```python
from build123d import *

# Parameters (mm, degrees)
SKETCH1_W               = 71
SKETCH1_H               = 70
SKETCH1_W_2             = 68
SKETCH1_H_2             = 67
BOSS_EXTRUDE1_DEPTH     = 17.2
BOSS_EXTRUDE2_START     = 17.2
SKETCH1_2_W             = 71
SKETCH1_2_H             = 70
BOSS_EXTRUDE2_DEPTH     = 1.5
CUT_EXTRUDE1_REACH      = 96.232
SKETCH6_W               = 5.15
SKETCH6_H               = 1.8
MIRROR2_COPY_1_REACH    = 96.232
MIRROR2_COPY_1_SKETCH_W = 5.15
MIRROR2_COPY_1_SKETCH_H = 1.8
CUT_EXTRUDE2_REACH      = 96.978
SKETCH7_W               = 9.92
SKETCH7_H               = 21.65
SKETCH8_R               = 2.15
SKETCH8_R_2             = 0.4
SKETCH8_W               = 1.5
SKETCH8_H               = 1.5
BOSS_EXTRUDE6_DEPTH     = 5.7


with BuildPart() as part:
    # Sketch1 → Boss-Extrude1 (new body)
    with BuildSketch(Plane.XY):
        with Locations((-24.75, 25.25)):
            Rectangle(SKETCH1_W, SKETCH1_H)
        with Locations((-24.75, 25.25)):
            Rectangle(SKETCH1_W_2, SKETCH1_H_2, mode=Mode.SUBTRACT)
    extrude(amount=BOSS_EXTRUDE1_DEPTH)

    # Sketch1<2> → Boss-Extrude2 (add)
    with BuildSketch(Plane.XY.offset(BOSS_EXTRUDE2_START)):
        with Locations((-24.75, 25.25)):
            Rectangle(SKETCH1_2_W, SKETCH1_2_H)
    extrude(amount=BOSS_EXTRUDE2_DEPTH)

    # Sketch6 → Cut-Extrude1 (cut, up to next)
    with BuildSketch(Plane(origin=(0, 60.25, 0), x_dir=(1, 0, 0), z_dir=(0, 1, 0)), mode=Mode.PRIVATE) as cut_extrude1_sk1:
        with Locations((6.675, -5.25)):
            Rectangle(SKETCH6_W, SKETCH6_H)
    cut_extrude1_tool1 = extrude(cut_extrude1_sk1.sketch, amount=-CUT_EXTRUDE1_REACH, mode=Mode.PRIVATE) & part.part
    cut_extrude1 = cut_extrude1_tool1.solids().sort_by_distance((6.675, 60.25, 5.25))[0]
    add(cut_extrude1, mode=Mode.SUBTRACT)

    # Mirror1: Cut-Extrude1 across plane
    add(cut_extrude1.mirror(Plane(origin=(-24.75, 0, 0), x_dir=(0, 0, 1), z_dir=(1, 0, 0))), mode=Mode.SUBTRACT)

    # Mirror2: Cut-Extrude1 across plane
    add(cut_extrude1.mirror(Plane.ZX.offset(25.25)), mode=Mode.SUBTRACT)

    # Mirror2 copy 1 sketch → Mirror2 copy 1 (cut, up to next)
    with BuildSketch(Plane(origin=(-49.5, -9.75, 0), x_dir=(-1, 0, 0), z_dir=(0, -1, 0)), mode=Mode.PRIVATE) as mirror2_copy_1_sk1:
        with Locations((6.675, -5.25)):
            Rectangle(MIRROR2_COPY_1_SKETCH_W, MIRROR2_COPY_1_SKETCH_H)
    mirror2_copy_1_tool1 = extrude(mirror2_copy_1_sk1.sketch, amount=-MIRROR2_COPY_1_REACH, mode=Mode.PRIVATE) & part.part
    add(mirror2_copy_1_tool1.solids().sort_by_distance((-56.175, -9.75, 5.25))[0], mode=Mode.SUBTRACT)

    # Sketch7 → Cut-Extrude2 (cut, up to next)
    with BuildSketch(Plane.ZY.offset(60.25), mode=Mode.PRIVATE) as cut_extrude2_sk1:
        with Locations((6.74, 22.95)):
            Rectangle(SKETCH7_W, SKETCH7_H)
    cut_extrude2_tool1 = extrude(cut_extrude2_sk1.sketch, amount=-CUT_EXTRUDE2_REACH, mode=Mode.PRIVATE) & part.part
    add(cut_extrude2_tool1.solids().sort_by_distance((-60.25, 22.95, 6.74))[0], mode=Mode.SUBTRACT)

    # Sketch8 → Boss-Extrude6 (add)
    # profile 1 of 4: a face of its own
    with BuildSketch(Plane(origin=(0, 0, 17.2), x_dir=(-1, 0, 0), z_dir=(0, 0, -1))):
        with Locations((51.65, 49.525)):
            Circle(SKETCH8_R)
        with Locations((51.65, 49.525)):
            Circle(SKETCH8_R_2, mode=Mode.SUBTRACT)
    # profile 2 of 4: a face of its own
    with BuildSketch(Plane(origin=(0, 0, 17.2), x_dir=(-1, 0, 0), z_dir=(0, 0, -1))):
        with Locations((-2.3, 49.625)):
            Circle(SKETCH8_R)
        with Locations((-2.3, 49.625)):
            Circle(SKETCH8_R_2, mode=Mode.SUBTRACT)
    # profile 3 of 4: a face of its own
    with BuildSketch(Plane(origin=(0, 0, 17.2), x_dir=(-1, 0, 0), z_dir=(0, 0, -1))):
        with Locations((-1.95, 1.075)):
            Circle(SKETCH8_R)
        with Locations((-1.95, 1.075)):
            Circle(SKETCH8_R_2, mode=Mode.SUBTRACT)
    # profile 4 of 4: a face of its own
    with BuildSketch(Plane(origin=(0, 0, 17.2), x_dir=(-1, 0, 0), z_dir=(0, 0, -1))):
        with Locations((53, -0.125)):
            Rectangle(SKETCH8_W, SKETCH8_H)
    extrude(amount=BOSS_EXTRUDE6_DEPTH)


solid = part.part
```
For this review, take the finished solid that the model builds, in its own axes (mm). A direction names the side the tool comes from. Coordinates: 2 decimals unless noted, no trailing zeros. Order: outer loops, then holes, each group sorted by start corner. A loop starts at its lowest first (then second) coordinate and runs counter-clockwise, first axis right, second up. Notation, with made-up numbers: (26, 49) -> (60, 49) arc R13 cw to (60, 67) -> close; hole circle Ø8 at (36, 75.5). An arc over 180 degrees is marked (long way). Answer as CSV lines item,"result".
Q1. We need section C-C (z = 14.75). Count the separate pieces of the cut face and the enclosed holes in it, plus the area to 3 significant figures.
Model answer:
separate pieces,"5"
enclosed holes,"4"
area,"458 mm2"
Q2. Draft analysis for pull direction Y (two halves, no side actions). For faces 3 (the face through (10.75, 25, 9)), 4 (the face through (2.5, 1.1, 11.5)), 5 (the face through (1.144, 51.438, 14.39)), 6 (the face through (-25, 60.25, 9)), state which applies: released by +Y, released by -Y, zero draft, split by the parting line, or undercut.
Model answer:
face 3,"zero draft"
face 4,"undercut"
face 5,"undercut"
face 6,"released by +Y"
Q3. Clearance check with flat-ended pins moving along their axes: pin 1 Ø20 at (x, y) = (-26, 20) entering from -Z; pin 2 Ø1.6 at (x, y) = (-52.5, 0) entering from -Z. State where each tip first meets the part, or that it passes through.
Model answer:
pin 1,"stops at z = 17.2"
pin 2,"stops at z = 11.5"
Q4. We need section A-A (x = -55). State the section outline as (y, z) points, plus the area to 3 significant figures.
Model answer:
outline,"(-9.75, 0) -> (-8.25, 0) -> (-8.25, 4.35) -> (-9.75, 4.35) -> close; (-9.75, 6.15) -> (-8.25, 6.15) -> (-8.25, 17.2) -> (58.75, 17.2) -> (58.75, 6.15) -> (60.25, 6.15) -> (60.25, 18.7) -> (-9.75, 18.7) -> close; (58.75, 0) -> (60.25, 0) -> (60.25, 4.35) -> (58.75, 4.35) -> close"
area,"151 mm2"
Q5. We need section B-B (y = 21). State the section outline as (x, z) points, plus the area to 3 significant figures.
Model answer:
outline,"(-60.25, 0) -> (-58.75, 0) -> (-58.75, 1.78) -> (-60.25, 1.78) -> close; (-60.25, 11.7) -> (-58.75, 11.7) -> (-58.75, 17.2) -> (9.25, 17.2) -> (9.25, 0) -> (10.75, 0) -> (10.75, 18.7) -> (-60.25, 18.7) -> close"
area,"143 mm2"
Q6. For faces 1 (the face through (-25, -9.75, 9)), 2 (the face through (2, 49, 11.5)), list the 3-axis set-ups (+Z, -Z, +X, -X, +Y, -Y) from which the entire face can be reached by the end or side of a thin tool; tool diameter is ignored.
Model answer:
face 1,"+Z, -Z, +X, -X, -Y"
face 2,"-Z"
Q7. We need section D-D (x = -8). State the section outline as (y, z) points.
Model answer:
outline,"(-9.75, 0) -> (-8.25, 0) -> (-8.25, 17.2) -> (58.75, 17.2) -> (58.75, 0) -> (60.25, 0) -> (60.25, 18.7) -> (-9.75, 18.7) -> close"
Q8. Wall thickness on line 1 along Y through (x, z) = (-6.5, 13); line 2 along X through (y, z) = (5.5, 3.25); line 3 along Z through (x, y) = (-13, 9.5): over which ranges is each line inside the solid? List them lowest first. Write a range as [from, to].
Model answer:
line 1,"y = [-9.75, -8.25], [58.75, 60.25]"
line 2,"x = [-60.25, -58.75], [9.25, 10.75]"
line 3,"z = [17.2, 18.7]"
